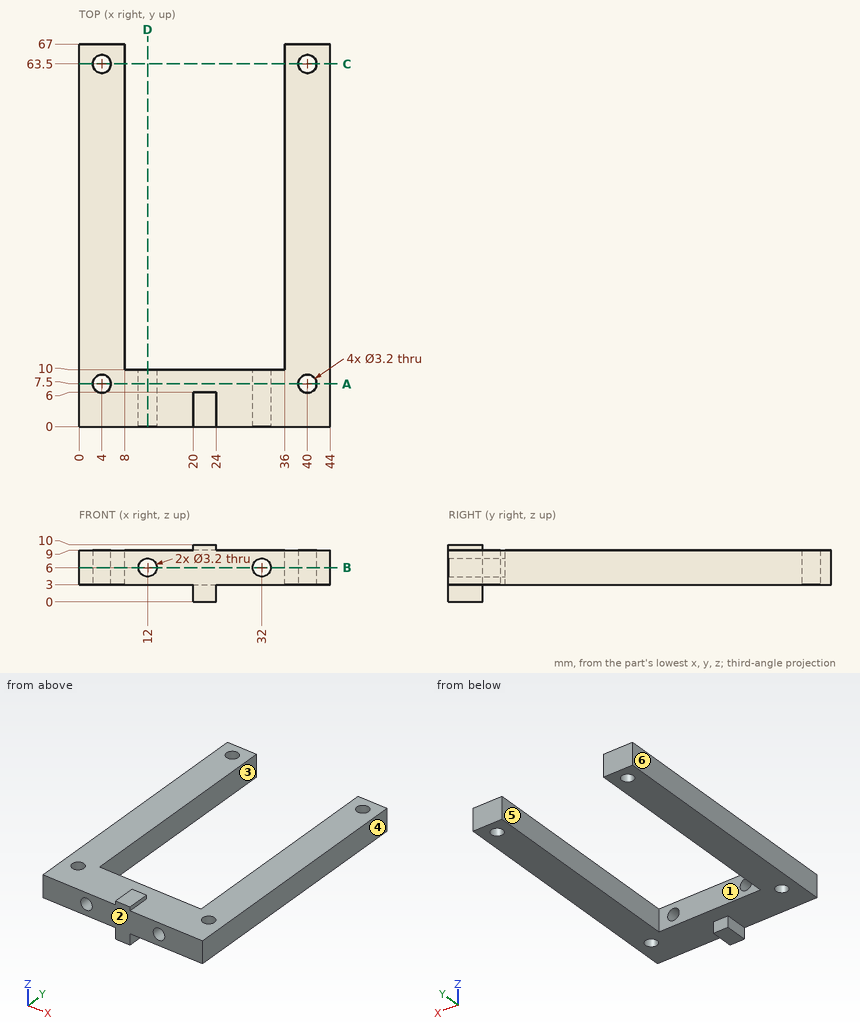
Job drawing, mm, ordinate dimensions from the low corner. One solid piece. A direction names the side the tool comes from. Round coordinates to 2 decimals unless told otherwise and drop trailing zeros. Write each loop counter-clockwise with the first axis right and the second up, starting at its lowest first coordinate (ties: lowest second). Pieces come first, ordered by that corner, then holes.
1) Band-saw the part on C-C, the plane y = 63.5. List the corners of the cut face in (x, z), and give its area (3 significant figures).
2) Mould opens along X. For the marked faces 1, 2, 3 and 4 say: +X half, -X half, draft (parallel to the pull), parting line (faces both ways), or undercut.
3) Band-saw the part on B-B, the plane z = 6. List the corners of the cut face in (x, y), and give its area (3 significant figures).
4) Band-saw the part on A-A, the plane y = 7.5. List the corners of the cut face in (x, z).
5) 3-axis set-ups, long thin cutter, end or side, ignore diameter. For the marked faces 5 and 6: which of +Z, -Z, +X, -X, +Y, -Y reach the whole face in a straight line?
6) Drill centre lines: probe 1 along X at (y, z) = (63.5, 4.6); probe 2 along Y at (x, z) = (40, 4.55); probe 3 along X at (y, z) = (4.25, 6). Where is each one in solid material? Low to high.
7) Band-saw the part on D-D, the plane x = 12. List the corners of the cut face in (y, z).
8) Pin check, flat tips, straight feed: pin 1 (5 mm diameter, centred on x = 6.5, y = 24, fed in from +Z); pin 2 (13 mm diameter, centred on x = 31, y = 19.5, fed in from -Z); pin 3 (1.5 mm diameter, centred on x = 21, z = 1.5, fed in from +Y); pin 4 (2.5 mm diameter, centred on x = 12, z = 6, fed in from +Y). Stop position of each tip, or through.
Ans:
1. outline: (0, 3) - (2.4, 3) - (2.4, 9) - (0, 9) - close; (5.6, 3) - (8, 3) - (8, 9) - (5.6, 9) - close; (36, 3) - (38.4, 3) - (38.4, 9) - (36, 9) - close; (41.6, 3) - (44, 3) - (44, 9) - (41.6, 9) - close
1. area: 57.6 mm2
2. face 1: undercut
2. face 2: draft
2. face 3: undercut
2. face 4: +X half
3. outline: (0, 0) - (10.4, 0) - (10.4, 10) - (8, 10) - (8, 67) - (0, 67) - close; (13.6, 0) - (30.4, 0) - (30.4, 10) - (13.6, 10) - close; (33.6, 0) - (44, 0) - (44, 67) - (36, 67) - (36, 10) - (33.6, 10) - close; hole circle Ø3.2 at (4, 7.5); hole circle Ø3.2 at (4, 63.5); hole circle Ø3.2 at (40, 7.5); hole circle Ø3.2 at (40, 63.5)
3. area: 1,260 mm2
4. outline: (0, 3) - (2.4, 3) - (2.4, 9) - (0, 9) - close; (5.6, 3) - (38.4, 3) - (38.4, 9) - (5.6, 9) - close; (41.6, 3) - (44, 3) - (44, 9) - (41.6, 9) - close; hole circle Ø3.2 at (12, 6); hole circle Ø3.2 at (32, 6)
5. face 5: +Z, -Z, +Y
5. face 6: +Z, -Z, -X, +Y, -Y
6. probe 1: x = 0 to 2.4, 5.6 to 8, 36 to 38.4, 41.6 to 44
6. probe 2: y = 0 to 5.9, 9.1 to 61.9, 65.1 to 67
6. probe 3: x = 0 to 10.4, 13.6 to 30.4, 33.6 to 44
7. outline: (0, 3) - (10, 3) - (10, 4.4) - (0, 4.4) - close; (0, 7.6) - (10, 7.6) - (10, 9) - (0, 9) - close
8. pin 1: stops at z = 9
8. pin 2: stops at z = 3
8. pin 3: stops at y = 6
8. pin 4: passes through
